Geometry check sheet. Reference: the model listing, model coordinates, mm. Face numbers are marked on the shaded views. Coordinates: 2 decimals unless noted, no trailing zeros. Order: outer loops, then holes, each group sorted by start corner. A loop starts at its lowest first (then second) coordinate and runs counter-clockwise, first axis right, second up.
```python
from build123d import *

# Parameters (mm, degrees)
F0_R     = 55
F0_R_2   = 51
F0_R_3   = 47
F1_DEPTH = 5
F2_DEPTH = 500
F3_DEPTH = 50
F4_R     = 10
F5_DEPTH = 25
F6_DEPTH = 25
F7_DEPTH = 25


# Not quite as in the source:
# - a fillet or chamfer that OpenCascade refuses, or shapes differently, is made with other operations: its cross-section is extruded or revolved along the edge and cut away or added


with BuildPart() as f1:
    # F0 (on Top) → F1 (new body)
    with BuildSketch(Plane.XY):
        Circle(F0_R)
        Circle(F0_R_2, mode=Mode.SUBTRACT)
        Circle(F0_R_2)
        Circle(F0_R_3, mode=Mode.SUBTRACT)
        Circle(F0_R_3)
    extrude(amount=F1_DEPTH)

    # F0 (on Top) → F2 (join)
    with BuildSketch(Plane.XY):
        Circle(F0_R_2)
        Circle(F0_R_3, mode=Mode.SUBTRACT)
    extrude(amount=F2_DEPTH)

    # F3 (add): a face of the model
    f3_faces = [f1.faces().sort_by_distance(p)[0] for p in [
        (-53.4443650814, 0, 5),
    ]]
    extrude(f3_faces, amount=F3_DEPTH)

    # F4
    f4_edges = [f1.edges().sort_by_distance(p)[0] for p in [
        (-55, 0, 0),
    ]]
    fillet(f4_edges, radius=F4_R)

    # F0 (on Top) → F5 (join)
    with BuildSketch(Plane.XY):
        Circle(F0_R)
        Circle(F0_R_2, mode=Mode.SUBTRACT)
    extrude(amount=F5_DEPTH)

    # F0 (on Top) → F6 (join)
    with BuildSketch(Plane.XY):
        Circle(F0_R)
        Circle(F0_R_2, mode=Mode.SUBTRACT)
    extrude(amount=F6_DEPTH)

    # F0 (on Top) → F7 (join)
    with BuildSketch(Plane.XY):
        Circle(F0_R)
        Circle(F0_R_2, mode=Mode.SUBTRACT)
    extrude(amount=F7_DEPTH)

    # F8: fillet of radius 7 on 1 edges, made by hand

    # F8_s1 → F8_t2 (revolve, cut)
    with BuildSketch(Plane.XZ):
        with BuildLine():
            ThreePointArc((55, 6.3245553203), (53.9160797831, 2.5828979336), (51, 0))
            Line((51, 0), (55, 0))
            Line((55, 0), (55, 6.3245553203))
        make_face()
    revolve(axis=Axis((0, 0, 0), (0, 0, 1)), mode=Mode.SUBTRACT)


solid = f1.part
```
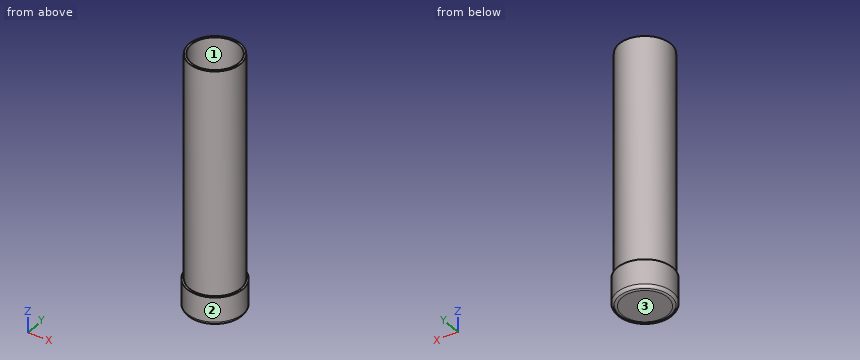
Item 1: Sectioned sample at D-D (z = 44.5). Record the cut outline in (x, y).
Item 2: Sectioned sample at A-A (x = 0). Record the cut outline in (y, z).
Item 3: Sectioned sample at C-C (z = 245). Record the cut outline in (x, y).
Item 4: Release check for a two-part mould opening along X. For the marked faces 1, 2 and 3 record: pulls with the +X half, pulls with the -X half, needs draft (parallel to the pull), parting line crosses it, or undercut.
Item 5: Thickness scan on line 1 along Y through (x, z) = (0, 407.5); line 2 along Y through (x, z) = (0, 1.35); line 3 along Z through (x, y) = (1.5, 39.5). Record the ranges inside material, lowest first.
Item 6: Depth check by flat-ended pin: P1, Ø8, axis at y = 8, z = 283, coming from the +X side; P2, Ø4, axis at y = 27.5, z = 296, coming from the -X side; P3, Ø3, axis at y = 33, z = 287.5, coming from the -X side. Enter the tip coordinate at first touch or a pass-through.
Geometry check:
1. outline: circle Ø110 at (0, 0); hole circle Ø94 at (0, 0)
2. outline: (-55, 6.32) arc R7 ccw to (-51, 0) - (-51, 2) arc R10 ccw to (-45, 0) - (45, 0) arc R10 ccw to (51, 2) - (51, 0) arc R7 ccw to (55, 6.32) - (55, 55) - (51, 55) - (51, 500) - (47, 500) - (47, 5) - (-47, 5) - (-47, 500) - (-51, 500) - (-51, 55) - (-55, 55) - close
3. outline: circle Ø102 at (0, 0); hole circle Ø94 at (0, 0)
4. face 1: undercut
4. face 2: parting line crosses it
4. face 3: needs draft
5. line 1: y = -51 to -47, 47 to 51
5. line 2: y = -52.92 to -51, -50.02 to 50.02, 51 to 52.92
5. line 3: z = 0 to 5
6. P1: stops at x = 50.84
6. P2: stops at x = -44.17
6. P3: stops at x = -40.11
